Design review of the part built by this model. Coordinates are the model's own, in mm. A direction names the side the tool comes from. Round coordinates to 2 decimals unless told otherwise and drop trailing zeros. Loops run counter-clockwise (first coordinate to the right, second up) from the corner with the lowest first, then second, coordinate; pieces in that order, holes last. Notation, with made-up numbers: (50.5, 15.25) - (101.5, 15.25) arc R24 cw to (101.5, 44.25) - close; hole circle Ø1 at (42.25, 65). An arc over 180 degrees is marked (long way). Return JSON: item names as keys, results as strings. Group by question number.
(1) For faces 1 (the flat face through (152.4, 130, 3)), 2 (the flat face through (0, 130, 3)), list the 3-axis set-ups (+Z, -Z, +X, -X, +Y, -Y) from which the entire face can be reached by the end or side of a thin tool; tool diameter is ignored.
(2) We need section B-B, the plane x = 39. Write out the cut boundary in (y, z), and give its area (3 significant figures).
(3) We need section C-C, the plane z = 8.5. Write out the cut boundary in (x, y) (3 decimals).
(4) Wall thickness on L1, parallel to X at y = 149.5, z = 3.5; L2, parallel to Y at x = 79.5, z = 1.25; L3, parallel to Y at x = 165.1, z = 4.75: over which ranges is each line inside the solid? List them lowest first. Write a range as [from, to].
(5) We need section A-A, the plane y = 46.5. Write out the cut boundary in (x, z).
(6) Clearance check with flat-ended pins moving along their axes: pin 1 (7 mm diameter, centred on y = 98.5, z = 4, fed in from -X); pin 2 (10 mm diameter, centred on x = 103, y = 33.5, fed in from +Z). State where each tip first meets the part, or that it passes through.
from build123d import *

# Parameters (mm, degrees)
F0_W     = 177.8
F0_H     = 263.2369608608
F1_DEPTH = 6.35
F2_W     = 63.5
F2_H     = 101.6
F3_DEPTH = 25
F5_D     = 5.1054
F6_DEPTH = 6.35


with BuildPart() as f1:
    # F0 (on Top) → F1 (new body)
    with BuildSketch(Plane.XY):
        with Locations((88.9, 131.6184804304)):
            Rectangle(F0_W, F0_H)
    extrude(amount=F1_DEPTH)

    # F2 (on face) → F3 (cut)
    with BuildSketch(Plane.XY.offset(6.35)):
        with Locations((57.15, 182.4184804304)):
            Rectangle(F2_W, F2_H)
        with Locations((57.15, 80.8184804304)):
            Rectangle(F2_W, F2_H)
        with Locations((120.65, 182.4184804304)):
            Rectangle(F2_W, F2_H)
        with Locations((120.65, 80.8184804304)):
            Rectangle(F2_W, F2_H)
    extrude(amount=-F3_DEPTH, mode=Mode.SUBTRACT)

    # F5 (through all)
    with Locations(Plane.XY.offset(6.35)):
        with Locations((12.7, 101.6184804304), (165.1, 101.6184804304)):
            Hole(F5_D / 2)

    # F4 (on face) → F6 (join)
    with BuildSketch(Plane.XY.offset(6.35)):
        with BuildLine():
            ThreePointArc((168.275, 117.4934804304), (167.3450640303, 119.7385444607), (165.1, 120.6684804304))
            Line((165.1, 120.6684804304), (165.1, 114.3184804304))
            ThreePointArc((165.1, 114.3184804304), (167.3450640303, 115.2484164001), (168.275, 117.4934804304))
        make_face()
        with BuildLine():
            Line((165.1, 114.3184804304), (165.1, 120.6684804304))
            ThreePointArc((165.1, 120.6684804304), (161.925, 117.4934804304), (165.1, 114.3184804304))
        make_face()
        with BuildLine():
            ThreePointArc((168.275, 85.7434804304), (167.3450640303, 87.9885444607), (165.1, 88.9184804304))
            Line((165.1, 88.9184804304), (165.1, 82.5684804304))
            ThreePointArc((165.1, 82.5684804304), (167.3450640303, 83.4984164001), (168.275, 85.7434804304))
        make_face()
        with BuildLine():
            Line((165.1, 82.5684804304), (165.1, 88.9184804304))
            ThreePointArc((165.1, 88.9184804304), (161.925, 85.7434804304), (165.1, 82.5684804304))
        make_face()
        with BuildLine():
            ThreePointArc((15.875, 85.7434804304), (14.9450640303, 87.9885444607), (12.7, 88.9184804304))
            Line((12.7, 88.9184804304), (12.7, 82.5684804304))
            ThreePointArc((12.7, 82.5684804304), (14.9450640303, 83.4984164001), (15.875, 85.7434804304))
        make_face()
        with BuildLine():
            Line((12.7, 82.5684804304), (12.7, 88.9184804304))
            ThreePointArc((12.7, 88.9184804304), (9.525, 85.7434804304), (12.7, 82.5684804304))
        make_face()
        with BuildLine():
            ThreePointArc((15.875, 117.4934804304), (14.9450640303, 119.7385444607), (12.7, 120.6684804304))
            Line((12.7, 120.6684804304), (12.7, 114.3184804304))
            ThreePointArc((12.7, 114.3184804304), (14.9450640303, 115.2484164001), (15.875, 117.4934804304))
        make_face()
        with BuildLine():
            Line((12.7, 114.3184804304), (12.7, 120.6684804304))
            ThreePointArc((12.7, 120.6684804304), (9.525, 117.4934804304), (12.7, 114.3184804304))
        make_face()
    extrude(amount=F6_DEPTH)


solid = f1.part
Solutions:
{
 "1": {"face 1": "+Z, -Z", "face 2": "+Z, -Z, -X, +Y, -Y"},
 "2": {"outline": "(0, 0) - (30.02, 0) - (30.02, 6.35) - (0, 6.35) - close; (233.22, 0) - (263.24, 0) - (263.24, 6.35) - (233.22, 6.35) - close", "area": "381 mm^2"},
 "3": {"outline": "circle Ø6.35 at (12.7, 85.743); circle Ø6.35 at (12.7, 117.493); circle Ø6.35 at (165.1, 85.743); circle Ø6.35 at (165.1, 117.493)"},
 "4": {"L1": "[0, 25.4], [152.4, 177.8]", "L2": "[0, 30.02], [233.22, 263.24]", "L3": "[0, 99.07], [104.17, 263.24]"},
 "5": {"outline": "(0, 0) - (25.4, 0) - (25.4, 6.35) - (0, 6.35) - close; (152.4, 0) - (177.8, 0) - (177.8, 6.35) - (152.4, 6.35) - close"},
 "6": {"pin 1": "x = 0", "pin 2": "z = 6.35"}
}
